The listing builds one solid part. Answer for the finished solid, in the listing's coordinates (mm). Face numbers are marked on the shaded views. A direction names the side the tool comes from. Coordinates: 2 decimals unless noted, no trailing zeros. Loops run counter-clockwise (first coordinate to the right, second up) from the corner with the lowest first, then second, coordinate; pieces in that order, holes last. Notation, with made-up numbers: (23, 69) - (28, 69) arc R24 ccw to (28, 90) - close; hole circle Ø8 at (33.25, 83). An arc over 180 degrees is marked (long way). Put each result on its own line as item: value.
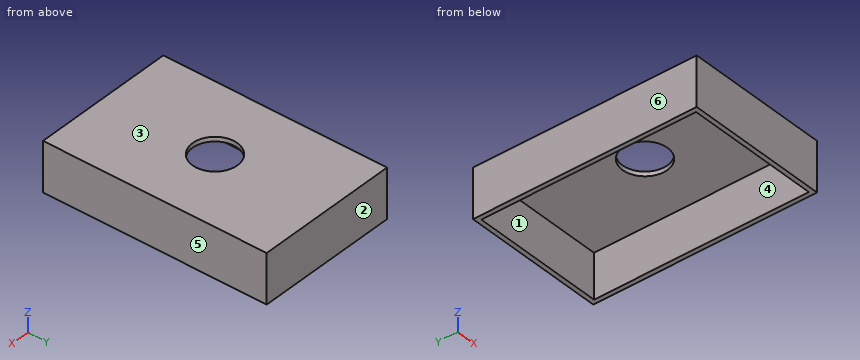
```python
from build123d import *

# Parameters (mm, degrees)
ESQUISSE1_W             = 160
ESQUISSE1_H             = 250
ESQUISSE1_W_2           = 150
ESQUISSE1_H_2           = 240
BOSS_EXTRU_1_DEPTH      = 50
ESQUISSE2_W             = 160
ESQUISSE2_H             = 250
BOSS_EXTRU_2_DEPTH      = 5
ESQUISSE4_R             = 25
ENL_V_MAT_EXTRU_1_DEPTH = 10


with BuildPart() as part:
    # Esquisse1 → Boss.-Extru.1 (new body)
    with BuildSketch(Plane.XY):
        with Locations((-80, 125)):
            Rectangle(ESQUISSE1_W, ESQUISSE1_H)
        with Locations((-80, 125)):
            Rectangle(ESQUISSE1_W_2, ESQUISSE1_H_2, mode=Mode.SUBTRACT)
    extrude(amount=BOSS_EXTRU_1_DEPTH)

    # Esquisse2 → Boss.-Extru.2 (add)
    with BuildSketch(Plane.XY.offset(50)):
        with Locations((-80, 125)):
            Rectangle(ESQUISSE2_W, ESQUISSE2_H)
    extrude(amount=BOSS_EXTRU_2_DEPTH)

    # Esquisse4 → Enlèv. mat.-Extru.1 (cut)
    with BuildSketch(Plane.XY.offset(55)):
        with Locations((-80, 125)):
            Circle(ESQUISSE4_R)
    extrude(amount=-ENL_V_MAT_EXTRU_1_DEPTH, mode=Mode.SUBTRACT)


solid = part.part
```
1) For a pull along X with two mould halves and no side action, classify the marked faces 3, 4, 5 and 6 as pulls with the +X half, pulls with the -X half, needs draft (parallel to the pull), parting line crosses it, or undercut.
Found:
face 3: needs draft
face 4: undercut
face 5: pulls with the +X half
face 6: pulls with the -X half
2) The part is cut by section D-D (x = -128.5). Give the vertices of the cut face in (y, z).
Found:
outline: (0, 0) - (5, 0) - (5, 50) - (245, 50) - (245, 0) - (250, 0) - (250, 55) - (0, 55) - close
3) This flat-tipped pin is pushed along its axis until it touches: pin 1 (1 mm diameter, centred on x = -80, y = 168, fed in from -Z). Where does it stop, or does it pass through?
Found:
pin 1: stops at z = 50
4) The part is cut by section B-B (y = 125). Give the vertices of the cut face in (x, z).
Found:
outline: (-160, 0) - (-155, 0) - (-155, 50) - (-105, 50) - (-105, 55) - (-160, 55) - close; (-55, 50) - (-5, 50) - (-5, 0) - (0, 0) - (0, 55) - (-55, 55) - close
5) The part is cut by section A-A (x = -80). Give the vertices of the cut face in (y, z).
Found:
outline: (0, 0) - (5, 0) - (5, 50) - (100, 50) - (100, 55) - (0, 55) - close; (150, 50) - (245, 50) - (245, 0) - (250, 0) - (250, 55) - (150, 55) - close
6) For the marked faces 1 and 2, determine the directions among +Z, -Z, +X, -X, +Y, -Y from which every point of the face is accessible in a straight line to the end or side of a thin tool.
Found:
face 1: -Z
face 2: +Z, -Z, +X, -X, +Y
7) Straight lines are drawn through the part: L1, parallel to Y at x = -73, z = 40; L2, parallel to Y at x = -80, z = 53; L3, parallel to X at y = 103.5, z = 31.5. For each, find the intervals that lie inside material, in ascending order. Write a range as [from, to].
Found:
L1: y = [0, 5], [245, 250]
L2: y = [0, 100], [150, 250]
L3: x = [-160, -155], [-5, 0]
8) The part is cut by section C-C (z = 45.5). Give the vertices of the cut face in (x, y), and give its area (3 significant figures).
Found:
outline: (-160, 0) - (0, 0) - (0, 250) - (-160, 250) - close; hole (-155, 5) - (-5, 5) - (-5, 245) - (-155, 245) - close
area: 4,000 mm^2
